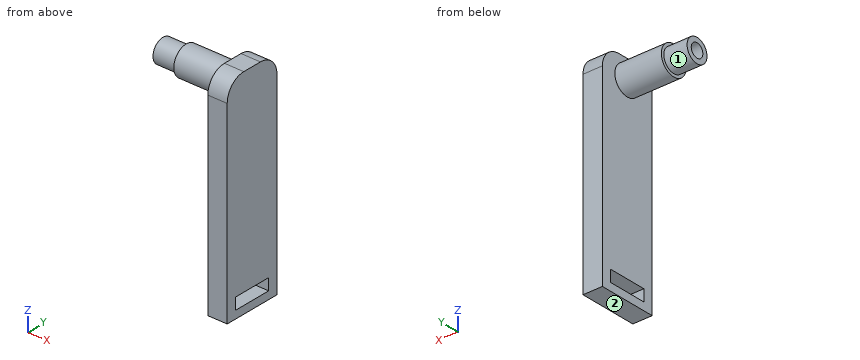
from build123d import *

# Parameters (mm, degrees)
SKETCH1_W           = 5
SKETCH1_H           = 55
BOSS_EXTRUDE1_DEPTH = 15
FILLET1_R           = 5
SKETCH2_W           = 3
SKETCH2_H           = 10
CUT_EXTRUDE1_DEPTH  = 5
SKETCH3_R           = 3.75
BOSS_EXTRUDE2_DEPTH = 12
SKETCH4_R           = 3
SKETCH4_R_2         = 1.75
BOSS_EXTRUDE3_DEPTH = 6


with BuildPart() as part:
    # Sketch1 → Boss-Extrude1 (new body)
    with BuildSketch(Plane(origin=(0, 0, 0), x_dir=(1, 0, 0), z_dir=(0, 1, 0))):
        with Locations((-59.380536913, 1.290268456)):
            Rectangle(SKETCH1_W, SKETCH1_H)
    extrude(amount=BOSS_EXTRUDE1_DEPTH)

    # Fillet1
    fillet1_edges = [part.edges().sort_by_distance(p)[0] for p in [
        (-59.380536913, 15, 26.209731544),
        (-59.380536913, 0, 26.209731544),
    ]]
    fillet(fillet1_edges, radius=FILLET1_R)

    # Sketch2 → Cut-Extrude1 (cut)
    with BuildSketch(Plane.ZY.offset(61.880536913)):
        with Locations((-25.290268456, 7.5)):
            Rectangle(SKETCH2_W, SKETCH2_H)
    extrude(amount=-CUT_EXTRUDE1_DEPTH, mode=Mode.SUBTRACT)

    # Sketch3 → Boss-Extrude2 (add)
    with BuildSketch(Plane.ZY.offset(61.880536913)):
        with Locations((21.209731544, 7.5)):
            Circle(SKETCH3_R)
    extrude(amount=BOSS_EXTRUDE2_DEPTH)

    # Sketch4 → Boss-Extrude3 (add)
    with BuildSketch(Plane.ZY.offset(73.880536913)):
        with Locations((21.209731544, 7.5)):
            Circle(SKETCH4_R)
        with Locations((21.209731544, 7.5)):
            Circle(SKETCH4_R_2, mode=Mode.SUBTRACT)
    extrude(amount=BOSS_EXTRUDE3_DEPTH)


solid = part.part
Input: part model. Units: mm. Frame: model coordinates. Face numbers are marked on the shaded views. A direction names the side the tool comes from. Round coordinates to 2 decimals unless told otherwise and drop trailing zeros. Loops run counter-clockwise (first coordinate to the right, second up) from the corner with the lowest first, then second, coordinate; pieces in that order, holes last. Notation, with made-up numbers: M 73.25,42.5 L 117.25,42.5 A26 cw 117.25,78.5 Z; hole C -1,82.25 d8. An arc over 180 degrees is marked long. Answer as CSV lines item,"result". Start each with the question number.
(1) Line query: line 1 (X direction, y = 13, z = -18); line 2 (Z direction, x = -59.5, y = 4.75); line 3 (Z direction, x = -68.75, y = 7.25). Output: solid intervals per line, ascending. Write a range as [from, to].
(2) Section D-D, the plane x = -68.5. Output: boundary loops of the cut face in (y, z).
(3) Section A-A, the plane y = 7.5. Output: boundary loops of the cut face in (x, z).
(4) Section C-C, the plane z = -9. Output: boundary loops of the cut face in (x, y).
(5) First-contact query: pin 1 (2 mm diameter, centred on y = 7.5, z = 21.21, fed in from -X). Flat tip, straight axial feed; report the tip coordinate or a pass-through.
(6) Section B-B, the plane x = -78. Output: boundary loops of the cut face in (y, z), plus the area to 3 significant figures.
(7) Reachability of the marked faces 1 and 2 from +Z, -Z, +X, -X, +Y, -Y: full face, straight path, thin tool, end or side. Return the list, or none.
Values found:
1,line 1,"x = [-61.88, -56.88]"
1,line 2,"z = [-28.79, -26.79], [-23.79, 26.2]"
1,line 3,"z = [17.47, 24.95]"
2,outline,"C 7.5,21.21 d7.5"
3,outline,"M -79.88,18.21 L -73.88,18.21 L -73.88,17.46 L -61.88,17.46 L -61.88,-23.79 L -56.88,-23.79 L -56.88,26.21 L -61.88,26.21 L -61.88,24.96 L -73.88,24.96 L -73.88,24.21 L -79.88,24.21 L -79.88,22.96 L -73.88,22.96 L -73.88,19.46 L -79.88,19.46 Z; M -61.88,-28.79 L -56.88,-28.79 L -56.88,-26.79 L -61.88,-26.79 Z"
4,outline,"M -61.88,0 L -56.88,0 L -56.88,15 L -61.88,15 Z"
5,pin 1,"stops at x = -73.88"
6,outline,"C 7.5,21.21 d6; hole C 7.5,21.21 d3.5"
6,area,"18.7 mm²"
7,face 1,"-X"
7,face 2,"-Z, +X, -X, +Y, -Y"
